Build history of the part. All positions in model axes, mm. Face numbers are marked on the shaded views. A direction names the side the tool comes from. Round coordinates to 2 decimals unless told otherwise and drop trailing zeros. Write each loop counter-clockwise with the first axis right and the second up, starting at its lowest first coordinate (ties: lowest second). Pieces come first, ordered by that corner, then holes.
1) Pull direction X, two halves, no side cores. Call the marked faces 5, 6 and 7: +X half, -X half, draft (parallel to the pull), parting line (faces both ways), or undercut.
2) Wall check: probe 1 along Y at (x, z) = (2, 22); probe 2 along Z at (x, y) = (-51, -32); probe 3 along X at (y, z) = (-29, 45). Give the ranges that are in metal, low to high.
3) Which spindle directions (+Z, -Z, +X, -X, +Y, -Y) get a long thin tool onto all of the face, cutting with end or side? Do the marked faces 1, 2, 3 and 4. Say none if no direction does.
4) Flat gauge pins, fed straight in: pin 1 (6 mm diameter, centred on x = -45, y = -19.5, fed in from -Z); pin 2 (9 mm diameter, centred on y = -19.5, z = 41.5, fed in from +X); pin 3 (15 mm diameter, centred on x = 10, z = 41.5, fed in from -Y); pin 4 (15 mm diameter, centred on y = -21, z = 33.5, fed in from -X). Where does each tip first touch, or does it go through?
5) Saw through at B-B (z = 44). Write the cut outline in (x, y).
6) Saw through at D-D (y = -8). Write the cut outline in (x, z).
7) Saw through at C-C (x = 0). Write the cut outline in (y, z), plus the area to 3 significant figures.
8) Saw through at A-A (y = -45). Write the cut outline in (x, z), plus the area to 3 significant figures.
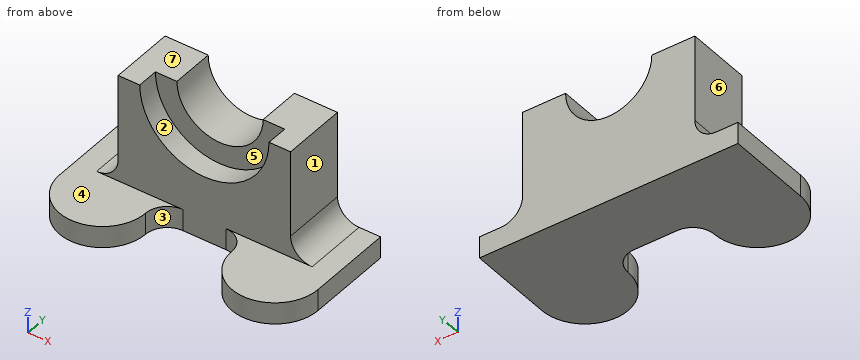
Autodesk Fusion 360 part; units mm, degrees
sketch "Sketch1" plane through (0, 0, 0) normal (0, 1, 0) x (1, 0, 0)
  line L0 (0, 0) -> (60, 0)
  line L1 (60, 0) -> (60, -10)
  line L2 (60, -10) -> (50, -10)
  line L3 (40, -20) -> (40, -60)
  line L4 (-40, -60) -> (-40, -20)
  line L5 (-50, -10) -> (-60, -10)
  line L6 (-60, -10) -> (-60, 0)
  line L7 (-60, 0) -> (0, 0)
  arc A0 (-40, -20) -> (-50, -10) centre (-50, -20) ccw
  arc A1 (50, -10) -> (40, -20) centre (50, -20) ccw
  arc A2 (20, -60) -> (-20, -60) centre (0, -60) ccw
  arc A3 (30, -60) -> (-30, -60) centre (0, -60) ccw
  line L8 (40, -60) -> (20, -60)
  line L9 (-20, -60) -> (-40, -60)
  dimension "d1" = 60
  dimension "d2" = 60
  dimension "d3" = 10
  dimension "d4" = 10
  dimension "d5" = 10
  dimension "d6" = 40
  dimension "d7" = 40
  dimension "d8" = 60
  dimension "d9" = 40
  dimension "d10" = 40
  dimension "d11" = 60
  dimension "d12" = 40
sketch "Sketch2" plane through (0, 0, 0) normal (0, 0, 1) x (1, 0, 0)
  line L0 (60, 0) -> (60, -40)
  line L1 (0, 0) -> (0, -30)
  line L2 (0, -30) -> (10, -30)
  arc A0 (20, -40) -> (60, -40) centre (40, -40) ccw
  line L3 (0, 0) -> (60, 0)
  arc A1 (20, -40) -> (10, -30) centre (10, -40) ccw
  dimension "d18" = 60
  dimension "d21" = 60
  dimension "d22" = 30
  dimension "d23" = 40
  dimension "d24" = 40
  dimension "d26" = 40
  dimension "d27" = 40
  dimension "d28" = 10
  dimension "d33" = 20
extrude "Extrude1" add sketch "Sketch1" against normal blind 30 contours L0 L1 L2 L3 L4 L5 L6 L7 A0 A1 A3 L8 L9
extrude "Extrude2" add sketch "Sketch1" against normal blind 20 contours A2 A3 L8 L9
extrude "Extrude3" add sketch "Sketch2" along normal blind 10
mirror "Mirror1" about plane through (0, 0, 0) normal (1, 0, 0) of "Extrude3"
equation "d9 = d6"
equation "d12 = d6"
Evaluation:
1. face 5: undercut
1. face 6: -X half
1. face 7: draft
2. probe 1: y = -30 to 0
2. probe 2: z = 0 to 10
2. probe 3: x = -40 to -25.98, 25.98 to 40
3. face 1: +Z, +X, +Y, -Y
3. face 2: +Z, -Y
3. face 3: +Z, -Z, -Y
3. face 4: +Z, -X, -Y
4. pin 1: stops at z = 0
4. pin 2: stops at x = 40
4. pin 3: stops at y = -20
4. pin 4: stops at x = -40
5. outline: (-40, -30) - (-25.38, -30) - (-25.38, -20) - (-12, -20) - (-12, 0) - (-40, 0) - close; (12, -20) - (25.38, -20) - (25.38, -30) - (40, -30) - (40, 0) - (12, 0) - close
6. outline: (-60, 0) - (60, 0) - (60, 10) - (50, 10) arc R10 cw to (40, 20) - (40, 60) - (20, 60) arc R20 cw to (-20, 60) - (-40, 60) - (-40, 20) arc R10 cw to (-50, 10) - (-60, 10) - close
7. outline: (-30, 0) - (0, 0) - (0, 40) - (-20, 40) - (-20, 30) - (-30, 30) - close
7. area: 1,100 mm2
8. outline: (-59.36, 0) - (-20.64, 0) - (-20.64, 10) - (-59.36, 10) - close; (20.64, 0) - (59.36, 0) - (59.36, 10) - (20.64, 10) - close
8. area: 775 mm2
